from build123d import *

# Parameters (mm, degrees)
F1_DEPTH      = 12.7
F2_W          = 508
F2_H          = 304.8
F2_W_2        = 355.6
F2_H_2        = 203.2
F3_DEPTH      = 6.35
F4_R          = 12.7
F5_W          = 76.2
F5_H          = 25.4
F6_DEPTH      = 3.81
F6_DEPTH_BACK = 25.4
F8_DEPTH      = 87.376
F9_W          = 63.5
F9_H          = 25.4
F10_DEPTH     = 3.81
F12_DEPTH     = 76.2


with BuildPart() as f1:
    # F0 (on Front) → F1 (new body, symmetric)
    with BuildSketch(Plane.XZ):
        Polygon((254, -17.3418857157), (203.2, -17.3418857157), (203.2, -127), (-203.2, -127), (-203.2, 127), (203.2, 127), (203.2, 14.4019788131), (241.3, 14.4019788131), (241.3, 127), (279.4, 127), (279.4, 152.4), (254, 152.4), (241.3, 152.4), (-228.6, 152.4), (-228.6, -152.4), (279.4, -152.4), (279.4, 105.8309227228), (254, 105.8309227228), (254, 0), align=None)
    extrude(amount=F1_DEPTH, both=True)

    # F2 (on face) → F3 (join)
    with BuildSketch(Plane.XZ.offset(12.7)):
        with Locations((25.4, 0)):
            Rectangle(F2_W, F2_H)
        Rectangle(F2_W_2, F2_H_2, mode=Mode.SUBTRACT)
    extrude(amount=F3_DEPTH)

    # F4
    f4_edges = [f1.edges().sort_by_distance(p)[0] for p in [
        (279.4, -3.175, -152.4),
        (-228.6, -3.175, -152.4),
        (-228.6, -3.175, 152.4),
        (279.4, -3.175, 152.4),
    ]]
    fillet(f4_edges, radius=F4_R)

    # F5 (on face) → F6 (join, two sides)
    with BuildSketch(Plane.XY.offset(-127)) as f6_sk:
        with Locations((-114.3, 0)):
            Rectangle(F5_W, F5_H)
    extrude(amount=F6_DEPTH)
    extrude(f6_sk.sketch, amount=-F6_DEPTH_BACK)

    # F7 (on face) → F8 (cut)
    with BuildSketch(Plane.YZ.offset(-76.2)):
        with BuildLine():
            add(Edge.make_bspline(
                [(12.7, -123.19), (10.5594976368, -123.19), (10.9031747427, -126.1164686911), (10.1332584811, -126.8581633475), (6.7809096129, -127)],
                knots=[0, 0, 0, 0, 0.2592828913, 0.6394583018, 0.6394583018, 0.6394583018, 0.6394583018], degree=3))
            Line((12.7, -123.19), (-12.7, -123.19))
            Line((-12.7, -123.19), (-12.7, -127))
            Line((-12.7, -127), (6.7809096129, -127))
        make_face()
    extrude(amount=-F8_DEPTH, mode=Mode.SUBTRACT)

    # F9 (on face) → F10 (join)
    with BuildSketch(Plane(origin=(0, 0, 127), x_dir=(1, 0, 0), z_dir=(0, 0, -1))):
        with Locations((120.65, 0)):
            Rectangle(F9_W, F9_H)
    extrude(amount=F10_DEPTH)

    # F11 (on face) → F12 (cut)
    with BuildSketch(Plane.YZ.offset(152.4)):
        with BuildLine():
            Line((-12.7, 123.19), (12.7, 123.19))
            add(Edge.make_bspline(
                [(12.7, 123.19), (10.4529513046, 123.19), (11.7430118211, 126.146945185), (9.7733114077, 126.8663682916), (5.5950677895, 127)],
                knots=[0, 0, 0, 0, 0.2484068186, 0.6533950313, 0.6533950313, 0.6533950313, 0.6533950313], degree=3))
            Line((5.5950677895, 127), (-12.7, 127))
            Line((-12.7, 127), (-12.7, 123.19))
        make_face()
    extrude(amount=-F12_DEPTH, mode=Mode.SUBTRACT)


solid = f1.part
Work out the finished part from the listing and answer in its coordinate system (mm). A direction names the side the tool comes from. Coordinates: 2 decimals unless noted, no trailing zeros. Write each loop counter-clockwise with the first axis right and the second up, starting at its lowest first coordinate (ties: lowest second). Pieces come first, ordered by that corner, then holes. Notation, with made-up numbers: M 52.25,-19.75 L 86.25,-19.75 A14 cw 86.25,-0.75 Z; hole C 49,-37 d7. An arc over 180 degrees is marked long. Write item = value, one per line.
1. Determine the mould class of faces 5 (the face through (-224.98, -3.4, -148.58)), 6 (the face through (241.3, 0, 70)), 7 (the face through (275.78, -2.95, 148.58)) for opening direction Z: released by +Z, released by -Z, zero draft, split by the parting line, or undercut.
Solution:
face_5 = released by -Z
face_6 = undercut
face_7 = released by +Z
2. The part is cut by section D-D (x = 193). Determine the outline of the cut face in (y, z).
Solution:
outline = M -19.05,-152.4 L 12.7,-152.4 L 12.7,-127 L -12.7,-127 L -12.7,127 L 12.7,127 L 12.7,152.4 L -19.05,152.4 Z
3. A flat-ended cylindrical pin translates along its axis: pin 1 (5 mm diameter, centred on y = -9.5, z = 111, fed in from +X). Find the tip coordinate at first contact, or state that the pin passes through.
Solution:
pin_1 = 241.3
4. For faces 1 (the face through (229, 0, -17.342)), 2 (the face through (-228.6, -3, -2)), 3 (the face through (267, 0, 105.831)), 4 (the face through (3, 0, -127)), determine the directions among +Z, -Z, +X, -X, +Y, -Y from which every point of the face is accessible in a straight line to the end or side of a thin tool.
Solution:
face_1 = +Y
face_2 = +Z, -Z, -X, +Y, -Y
face_3 = +X, +Y
face_4 = none
5. The part is cut by section B-B (x = 75). Determine the outline of the cut face in (y, z), then the cut area to 3 significant figures.
Solution:
outline = M -19.05,-152.4 L 12.7,-152.4 L 12.7,-127 L -12.7,-127 L -12.7,-101.6 L -19.05,-101.6 Z; M -19.05,101.6 L -12.7,101.6 L -12.7,127 L 12.7,127 L 12.7,152.4 L -19.05,152.4 Z
area = 1,940 mm2
6. Straight lines are drawn through the part: line 1 (X direction, y = -0.5, z = 88); line 2 (Z direction, x = -132, y = -11); line 3 (X direction, y = 10, z = -64). For each, find the intervals that lie inside material, in ascending order. Write a range as from..to.
Solution:
line_1 = -228.6..-203.2, 203.2..241.3, 254..279.4
line_2 = -152.4..-127, 127..152.4
line_3 = -228.6..-203.2, 203.2..279.4
7. The part is cut by section C-C (y = -7). Determine the outline of the cut face in (x, z), then the cut area to 3 significant figures.
Solution:
outline = M -228.6,-139.7 A12.7 ccw -215.9,-152.4 L 266.7,-152.4 A12.7 ccw 279.4,-139.7 L 279.4,105.83 L 254,105.83 L 254,-17.34 L 203.2,-17.34 L 203.2,-127 L -203.2,-127 L -203.2,127 L 203.2,127 L 203.2,14.4 L 241.3,14.4 L 241.3,127 L 279.4,127 L 279.4,139.7 A12.7 ccw 266.7,152.4 L -215.9,152.4 A12.7 ccw -228.6,139.7 Z
area = 47,900 mm2
8. The part is cut by section A-A (z = -82.5). Determine the outline of the cut face in (x, y), then the cut area to 3 significant figures.
Solution:
outline = M -228.6,-19.05 L -177.8,-19.05 L -177.8,-12.7 L -203.2,-12.7 L -203.2,12.7 L -228.6,12.7 Z; M 177.8,-19.05 L 279.4,-19.05 L 279.4,12.7 L 203.2,12.7 L 203.2,-12.7 L 177.8,-12.7 Z
area = 3,550 mm2
